Geometry: final body of the model. Coordinates: model frame, mm. A direction names the side the tool comes from. Round coordinates to 2 decimals unless told otherwise and drop trailing zeros. Loops run counter-clockwise (first coordinate to the right, second up) from the corner with the lowest first, then second, coordinate; pieces in that order, holes last. Notation, with made-up numbers: (-22.5, 57.25) - (-13.5, 57.25) arc R13 cw to (-13.5, 74.25) - close; hole circle Ø8 at (45, -17.5). An arc over 180 degrees is marked (long way). Answer in a Markdown table with one row per item. Add a question column.
from build123d import *

# Parameters (mm, degrees)
SKETCH6_W = 44.45
SKETCH6_H = 3.175


with BuildPart() as part:
    # Sweep1: sweep along a path in Sketch1
    with BuildLine(Plane(origin=(0, 0, 0), x_dir=(1, 0, 0), z_dir=(0, 1, 0))) as sweep1_path:
        Line((0, 0), (0, 123.825))
        ThreePointArc((0, 123.825), (7.439487758, 141.785512242), (25.4, 149.225))
        Line((25.4, 149.225), (35.9918, 149.225))
        ThreePointArc((35.9918, 149.225), (53.952312242, 141.785512242), (61.3918, 123.825))
        Line((61.3918, 123.825), (61.3918, 50.8))
        ThreePointArc((61.3918, 50.8), (68.831287758, 32.839487758), (86.7918, 25.4))
        Line((86.7918, 25.4), (97.3836, 25.4))
        ThreePointArc((97.3836, 25.4), (115.344112242, 32.839487758), (122.7836, 50.8))
        Line((122.7836, 50.8), (122.7836, 123.825))
        ThreePointArc((122.7836, 123.825), (130.223087758, 141.785512242), (148.1836, 149.225))
        Line((148.1836, 149.225), (158.7754, 149.225))
        ThreePointArc((158.7754, 149.225), (176.735912242, 141.785512242), (184.1754, 123.825))
        Line((184.1754, 123.825), (184.1754, 0))
    # Sketch6 → Sweep1 (sweep)
    with BuildSketch(Plane.XY):
        with Locations((0, -11.1125)):
            Rectangle(SKETCH6_W, SKETCH6_H)
    sweep(path=sweep1_path.line)


solid = part.part
1) Contact query for flat-ended pins moving along their axis: pin 1 Ø1 at (x, y) = (93, -11.5) entering from +Z (3 decimals); pin 2 Ø1.6 at (x, y) = (153.5, -11.5) entering from +Z. Output: stop coordinate, or through.
2) Pull-direction query (X, two-part tool) for faces 4 (the cylindrical face through (-8.644, -11.135, -157.129)), 5 (the cylindrical face through (130.69, -11.09, -16.76)), 6 (the flat face through (116, -12.7, -87)); classes: pulls with the +X half, pulls with the -X half, needs draft (parallel to the pull), parting line crosses it, or undercut.
3) Section A-A, the plane z = -96.5. Return the cut outline in (x, y) (3 decimals), and give its area (3 significant figures).
4) Section B-B, the plane y = -12.15. Return the cut outline in (x, z) (3 decimals), and give its area (3 significant figures).
5) Section D-D, the plane x = 109.5. Return the cut outline in (y, z) (3 decimals), and give its area (3 significant figures).
6) Section C-C, the plane z = -135.5. Return the cut outline in (x, y) (3 decimals), and give its area (3 significant figures).
7) Reachability of faces 1 (the cylindrical face through (69.295, -11.135, -157.869)), 2 (the flat face through (119, -9.525, -87)), 3 (the cylindrical face through (52.748, -11.09, -17.496)) from +Z, -Z, +X, -X, +Y, -Y: full face, straight path, thin tool, end or side. Return the list, or none.
8) Material intervals for line 1 along X through (y, z) = (-12.45, -66.5) (3 decimals); line 2 along X through (y, z) = (-11.85, -21) (3 decimals); line 3 along X through (y, z) = (-10.1, -10.5) (3 decimals), sorted ascending. Write a range as from..to.
Evaluation:
| question | item | result |
|---|---|---|
| 1 | pin 1 | stops at z = -3.175 |
| 1 | pin 2 | stops at z = -127 |
| 2 | face 4 | pulls with the -X half |
| 2 | face 5 | undercut |
| 2 | face 6 | needs draft |
| 3 | outline | (-22.225, -12.7) - (22.225, -12.7) - (22.225, -9.525) - (-22.225, -9.525) - close; (39.167, -12.7) - (83.617, -12.7) - (83.617, -9.525) - (39.167, -9.525) - close; (100.559, -12.7) - (145.009, -12.7) - (145.009, -9.525) - (100.559, -9.525) - close; (161.95, -12.7) - (206.4, -12.7) - (206.4, -9.525) - (161.95, -9.525) - close |
| 3 | area | 565 mm² |
| 4 | outline | (-22.225, -123.825) arc R47.625 ccw to (25.4, -171.45) - (35.992, -171.45) arc R47.625 ccw to (83.617, -123.825) - (83.617, -50.8) arc R3.175 cw to (86.792, -47.625) - (97.384, -47.625) arc R3.175 cw to (100.559, -50.8) - (100.559, -123.825) arc R47.625 ccw to (148.184, -171.45) - (158.775, -171.45) arc R47.625 ccw to (206.4, -123.825) - (206.4, 0) - (161.95, 0) - (161.95, -123.825) arc R3.175 cw to (158.775, -127) - (148.184, -127) arc R3.175 cw to (145.009, -123.825) - (145.009, -50.8) arc R47.625 ccw to (97.384, -3.175) - (86.792, -3.175) arc R47.625 ccw to (39.167, -50.8) - (39.167, -123.825) arc R3.175 cw to (35.992, -127) - (25.4, -127) arc R3.175 cw to (22.225, -123.825) - (22.225, 0) - (-22.225, 0) - close |
| 4 | area | 29,600 mm² |
| 5 | outline | (-12.7, -151.605) - (-9.525, -151.605) - (-9.525, -4.742) - (-12.7, -4.742) - close |
| 5 | area | 466 mm² |
| 6 | outline | (-20.772, -12.7) - (82.164, -12.7) - (82.164, -9.525) - (-20.772, -9.525) - close; (102.012, -12.7) - (204.947, -12.7) - (204.947, -9.525) - (102.012, -9.525) - close |
| 6 | area | 654 mm² |
| 7 | face 1 | -Z, +Y, -Y |
| 7 | face 2 | +Z, -Z, +X, -X, +Y |
| 7 | face 3 | +Z, +Y, -Y |
| 8 | line 1 | x = -22.225..22.225, 39.167..83.617, 100.559..145.009, 161.95..206.4 |
| 8 | line 2 | x = -22.225..22.225, 49.642..134.533, 161.95..206.4 |
| 8 | line 3 | x = -22.225..22.225, 61.414..122.762, 161.95..206.4 |
